The drawing under review shows one solid part. Ordinate dimensions are in mm from its lowest x, y, z. Give positions to 0.01 mm unless a question says otherwise; leave off trailing zeros. Order: outer loops, then holes, each group sorted by start corner. A loop starts at its lowest first (then second) coordinate and runs counter-clockwise, first axis right, second up. Notation, with made-up numbers: (-7.5, -26.5) - (12.5, -26.5) arc R16 cw to (12.5, -18.5) - close; hole circle Ø1 at (3, -8). An arc over 180 degrees is marked (long way). Use CSV: the item, a comma, the result in double quotes.
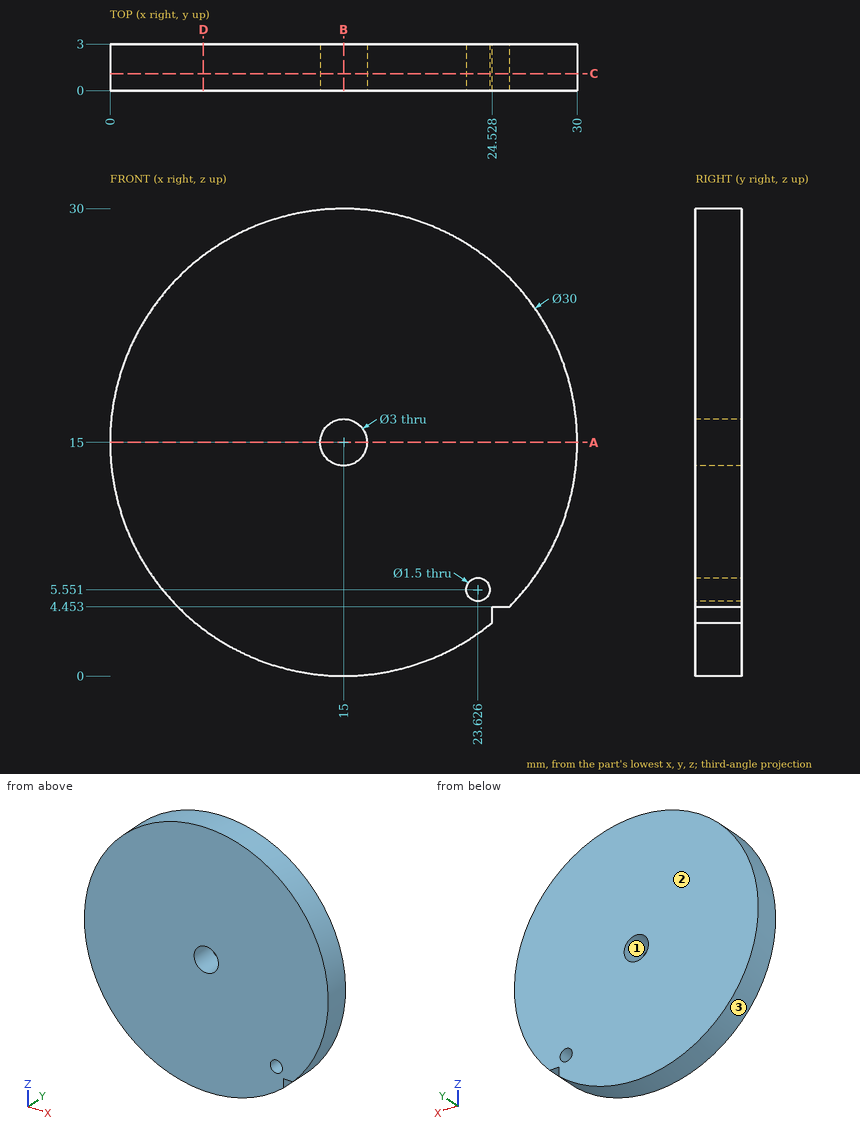
Item 1: Wall thickness on L1, parallel to X at y = 0.95, z = 15; L2, parallel to Z at x = 16, y = 2.85 (1 decimal); L3, parallel to X at y = 2.4, z = 12.5: over which ranges is each line inside the solid? List them lowest first.
Results list:
L1,"x = 0 to 13.5, 16.5 to 30"
L2,"z = 0 to 13.9, 16.1 to 30"
L3,"x = 0.21 to 29.79"
Item 2: Mouldability with a two-part tool opening along Z and no side actions: class the marked faces 1, 2 and 3 as pulls with the +Z half, pulls with the -Z half, needs draft (parallel to the pull), parting line crosses it, or undercut.
Results list:
face 1,"undercut"
face 2,"needs draft"
face 3,"parting line crosses it"
Item 3: Take a section at B-B, the plane x = 15. Give the boundary of the cut face in (y, z).
Results list:
outline,"(0, 0) - (3, 0) - (3, 13.5) - (0, 13.5) - close; (0, 16.5) - (3, 16.5) - (3, 30) - (0, 30) - close"
Item 4: Take a section at A-A, the plane z = 15. Give the boundary of the cut face in (x, y).
Results list:
outline,"(0, 0) - (13.5, 0) - (13.5, 3) - (0, 3) - close; (16.5, 0) - (30, 0) - (30, 3) - (16.5, 3) - close"
Item 5: Take a section at C-C, the plane y = 1.1. State how many separate pieces and enclosed holes the cut face has.
Results list:
separate pieces,"1"
enclosed holes,"2"
Item 6: Take a section at D-D, the plane x = 6. Give the boundary of the cut face in (y, z).
Results list:
outline,"(0, 3) - (3, 3) - (3, 27) - (0, 27) - close"
Item 7: Clearance check with flat-ended pins moving along their axes: pin 1 (1.5 mm diameter, centred on x = 18, y = 2.5, fed in from +Z); pin 2 (1.2 mm diameter, centred on x = 23.63, z = 5.55, fed in from +Y); pin 3 (0.5 mm diameter, centred on y = 1.5, z = 4, fed in from +X); pin 4 (1.5 mm diameter, centred on y = 1.5, z = 25, fed in from -X). State where each tip first meets the part, or that it passes through.
Results list:
pin 1,"stops at z = 29.83"
pin 2,"passes through"
pin 3,"stops at x = 24.53"
pin 4,"stops at x = 3.19"
